```python
from build123d import *

# Parameters (mm, degrees)
SKETCH1_W           = 120
SKETCH1_H           = 120
BOSS_EXTRUDE1_DEPTH = 40
CHAMFER1_SIZE       = 10
FILLET1_R           = 10
SHELL1_START        = -26.488905171
SHELL1_DEPTH        = 100
SHELL1_START_2      = 5
SHELL1_2_DEPTH      = 102


with BuildPart() as part:
    # Sketch1 → Boss-Extrude1 (new body)
    with BuildSketch(Plane.XY):
        with Locations((23.511094829, 55.943688507)):
            Rectangle(SKETCH1_W, SKETCH1_H)
    extrude(amount=BOSS_EXTRUDE1_DEPTH)

    # Chamfer1
    chamfer1_edges = [part.edges().sort_by_distance(p)[0] for p in [
        (83.511094829, 55.943688507, 40),
        (23.511094829, 115.943688507, 40),
        (-36.488905171, 55.943688507, 40),
        (23.511094829, -4.056311493, 40),
    ]]
    chamfer(chamfer1_edges, length=CHAMFER1_SIZE)

    # Fillet1
    fillet1_edges = [part.edges().sort_by_distance(p)[0] for p in [
        (-26.488905171, 55.943688507, 40),
        (23.511094829, 105.943688507, 40),
        (73.511094829, 55.943688507, 40),
        (23.511094829, 5.943688507, 40),
        (23.511094829, -4.056311493, 30),
        (83.511094829, 55.943688507, 30),
        (23.511094829, 115.943688507, 30),
        (-36.488905171, 55.943688507, 30),
    ]]
    fillet(fillet1_edges, radius=FILLET1_R)

    # Shell1: read off the stored shape, not the designer's step
    # Shell1 outline → Shell1 (cut)
    with BuildSketch(Plane.YZ.offset(SHELL1_START)):
        Polygon((5.943688507, 25.857864376), (5.943688507, 0), (105.943688507, 0), (105.943688507, 25.857864376), (101.801552884, 30), (10.085824131, 30), align=None)
    extrude(amount=SHELL1_DEPTH, mode=Mode.SUBTRACT)

    # Shell1 2 outline → Shell1 2 (add)
    with BuildSketch(Plane(origin=(0, 0, 0), x_dir=(1, 0, 0), z_dir=(0, 1, 0)).offset(SHELL1_START_2)):
        Polygon((73.511094829, -25.857864376), (69.368959206, -30), (73.511094829, -30), align=None)
        Polygon((-22.346769547, -30), (-26.488905171, -25.857864376), (-26.488905171, -30), align=None)
    extrude(amount=SHELL1_2_DEPTH)


solid = part.part
```
Build history of the part. All positions in model axes, mm. A direction names the side the tool comes from. Give positions to 0.01 mm unless a question says otherwise; leave off trailing zeros. Loops run counter-clockwise (first coordinate to the right, second up) from the corner with the lowest first, then second, coordinate; pieces in that order, holes last.
1) Probe line 1 along X through (y, z) = (99.5, 23); line 2 along Y through (x, z) = (8, 6.5); line 3 along Z through (x, y) = (57, 26). List the from-to ranges inside material, lowest first.
Values follow:
line 1: x = -36.49 to -26.49, 73.51 to 83.51
line 2: y = -4.06 to 5.94, 105.94 to 115.94
line 3: z = 30 to 40
2) Band-saw the part on A-A on z = 5. List the corners of the cut face in (x, y).
Values follow:
outline: (-36.49, -4.06) - (83.51, -4.06) - (83.51, 115.94) - (-36.49, 115.94) - close; hole (-26.49, 5.94) - (73.51, 5.94) - (73.51, 105.94) - (-26.49, 105.94) - close
3) Band-saw the part on C-C on y = 80.5. List the corners of the cut face in (x, z).
Values follow:
outline: (-36.49, 0) - (-26.49, 0) - (-26.49, 25.86) - (-22.35, 30) - (69.37, 30) - (73.51, 25.86) - (73.51, 0) - (83.51, 0) - (83.51, 25.86) arc R10 ccw to (80.58, 32.93) - (76.44, 37.07) arc R10 ccw to (69.37, 40) - (-22.35, 40) arc R10 ccw to (-29.42, 37.07) - (-33.56, 32.93) arc R10 ccw to (-36.49, 25.86) - close
4) Two-plate mould, pull along Y, no slides. Class faces 3 (the face through (-26.489, 55, 13)), 4 (the face through (-31, 57, 0)), 5 (the face through (23, -4.056, 13)), 6 (the face through (23, 105.944, 13)): released by +Y, released by -Y, zero draft, split by the parting line, or undercut.
Values follow:
face 3: undercut
face 4: zero draft
face 5: released by -Y
face 6: undercut
5) Band-saw the part on B-B on x = -15.5. List the corners of the cut face in (y, z), then the cut area to 3 significant figures.
Values follow:
outline: (-4.06, 0) - (5.94, 0) - (5.94, 25.86) - (10.09, 30) - (101.8, 30) - (105.94, 25.86) - (105.94, 0) - (115.94, 0) - (115.94, 25.86) arc R10 ccw to (113.01, 32.93) - (108.87, 37.07) arc R10 ccw to (101.8, 40) - (10.09, 40) arc R10 ccw to (3.01, 37.07) - (-1.13, 32.93) arc R10 ccw to (-4.06, 25.86) - close
area: 1,710 mm2
6) Band-saw the part on D-D on x = 75. List the corners of the cut face in (y, z), then the cut area to 3 significant figures.
Values follow:
outline: (-4.06, 0) - (115.94, 0) - (115.94, 25.86) arc R10 ccw to (113.01, 32.93) - (108.87, 37.07) arc R10 ccw to (107.43, 38.26) - (4.45, 38.26) arc R10 ccw to (3.01, 37.07) - (-1.13, 32.93) arc R10 ccw to (-4.06, 25.86) - close
area: 4,520 mm2
7) Drop flat-ended pins along their axis: P1, Ø2, axis at x = -13, y = 67, coming from the -Z side; P2, Ø2, axis at x = 17.5, z = 29.5, coming from the +Y side. Give the stop position or say it passes through.
Values follow:
P1: stops at z = 30
P2: stops at y = 115.59
8) 3-axis set-ups, long thin cutter, end or side, ignore diameter. For faces 1 (the face through (24.25, 105.58, 39.26)), 2 (the face through (23, 57, 30)): which of +Z, -Z, +X, -X, +Y, -Y reach the whole face in a straight line?
Values follow:
face 1: +Z, +X, -X, +Y
face 2: -Z
